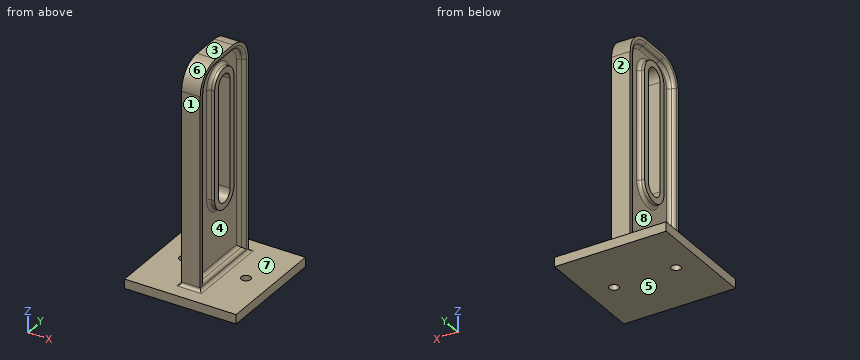
from build123d import *

# Parameters (mm, degrees)
SKETCH1_W           = 36
SKETCH1_H           = 36
BOSS_EXTRUDE1_DEPTH = 1.5
SKETCH2_R           = 1.5
CUT_EXTRUDE1_DEPTH  = 26.632011236
SKETCH3_W           = 6
SKETCH3_H           = 25
BOSS_EXTRUDE2_DEPTH = 70
CUT_EXTRUDE2_DEPTH  = 77.66322456
FILLET1_R           = 8
CUT_EXTRUDE3_DEPTH  = 2
FILLET4_R           = 1


with BuildPart() as part:
    # Sketch1 → Boss-Extrude1 (new, symmetric)
    with BuildSketch(Plane.XY):
        Rectangle(SKETCH1_W, SKETCH1_H)
    extrude(amount=BOSS_EXTRUDE1_DEPTH, both=True)

    # Sketch2 → Cut-Extrude1 (cut, through all)
    with BuildSketch(Plane.XY.offset(1.5)):
        with Locations((-10, 0)):
            Circle(SKETCH2_R)
        with Locations((10, 0)):
            Circle(SKETCH2_R)
    extrude(amount=-CUT_EXTRUDE1_DEPTH, mode=Mode.SUBTRACT)

    # Sketch3 → Boss-Extrude2 (add)
    with BuildSketch(Plane.XY.offset(1.5)):
        Rectangle(SKETCH3_W, SKETCH3_H)
    extrude(amount=BOSS_EXTRUDE2_DEPTH)

    # Sketch4 → Cut-Extrude2 (cut, through all)
    with BuildSketch(Plane(origin=(3, 0, 0), x_dir=(0, 0, -1), z_dir=(1, 0, 0))):
        with BuildLine():
            Line((-61.5, 3), (-26.5, 3))
            ThreePointArc((-26.5, 3), (-23.5, 0), (-26.5, -3))
            Line((-26.5, -3), (-61.5, -3))
            ThreePointArc((-61.5, -3), (-64.5, 0), (-61.5, 3))
        make_face()
    extrude(amount=-CUT_EXTRUDE2_DEPTH, mode=Mode.SUBTRACT)

    # Fillet1
    fillet1_edges = [part.edges().sort_by_distance(p)[0] for p in [
        (0, 12.5, 71.5),
        (0, -12.5, 71.5),
    ]]
    fillet(fillet1_edges, radius=FILLET1_R)

    # Sketch5 → Cut-Extrude3 (cut)
    with BuildSketch(Plane(origin=(3, 0, 0), x_dir=(0, 0, -1), z_dir=(1, 0, 0))):
        with BuildLine():
            Line((-3.5, -10.5), (-3.5, 10.5))
            Line((-3.5, 10.5), (-63.5, 10.5))
            ThreePointArc((-63.5, 10.5), (-67.742640687, 8.742640687), (-69.5, 4.5))
            Line((-69.5, 4.5), (-69.5, -4.5))
            ThreePointArc((-69.5, -4.5), (-67.742640687, -8.742640687), (-63.5, -10.5))
            Line((-63.5, -10.5), (-3.5, -10.5))
        make_face()
        with BuildLine():
            Line((-26.5, 5), (-61.5, 5))
            ThreePointArc((-61.5, 5), (-66.5, 0), (-61.5, -5))
            Line((-61.5, -5), (-26.5, -5))
            ThreePointArc((-26.5, -5), (-21.5, 0), (-26.5, 5))
        make_face(mode=Mode.SUBTRACT)
    cut_extrude3 = extrude(amount=-CUT_EXTRUDE3_DEPTH, mode=Mode.SUBTRACT)

    # Mirror1: Cut-Extrude3 across plane
    add(cut_extrude3.mirror(Plane(origin=(0, 0, 0), x_dir=(0, 0, 1), z_dir=(1, 0, 0))), mode=Mode.SUBTRACT)

    # Fillet4
    fillet4_edges = [part.edges().sort_by_distance(p)[0] for p in [
        (-3, -10.5, 33.5),
        (-3, -8.742640687, 67.742640687),
        (-3, 0, 69.5),
        (-3, 8.742640687, 67.742640687),
        (3, 10.5, 33.5),
        (3, 8.742640687, 67.742640687),
        (3, 0, 69.5),
        (3, -8.742640687, 67.742640687),
        (-1, 10.5, 33.5),
        (-1, 8.742640687, 67.742640687),
        (-1, 0, 69.5),
        (-1, -8.742640687, 67.742640687),
        (-1, -5, 44),
        (-1, 0, 66.5),
        (-1, 5, 44),
        (1, 10.5, 33.5),
        (1, 8.742640687, 67.742640687),
        (1, 0, 69.5),
        (1, -8.742640687, 67.742640687),
        (1, 0, 21.5),
        (1, -5, 44),
        (1, 0, 66.5),
        (0, 12.5, 1.5),
        (0, -12.5, 1.5),
        (-3, 0, 1.5),
        (3, 0, 1.5),
        (-3, 10.5, 33.5),
        (-3, 0, 3.5),
        (3, 0, 3.5),
        (3, -10.5, 33.5),
        (-1, 0, 3.5),
        (-1, -10.5, 33.5),
        (-1, 0, 21.5),
        (1, 0, 3.5),
        (1, -10.5, 33.5),
        (1, 5, 44),
    ]]
    fillet(fillet4_edges, radius=FILLET4_R - 0.0001)  # a hair under: the kernel refuses the full size


solid = part.part
Could you check a few things on this model? Use its own coordinates, in mm. Face numbers are marked on the shaded views. A direction names the side the tool comes from. Give positions to 0.01 mm unless a question says otherwise; leave off trailing zeros. Order: outer loops, then holes, each group sorted by start corner. A loop starts at its lowest first (then second) coordinate and runs counter-clockwise, first axis right, second up. Notation, with made-up numbers: (84.25, 7) - (105.25, 7) arc R23 cw to (105.25, 31) - close; hole circle Ø7 at (1, -30.5). An arc over 180 degrees is marked (long way). One line per item, written item: value. Start each with the question number.
1. Thinking about a two-plate mould opening in Y: for the marked faces 6, 7 and 8, which applies, +Y half, -Y half, draft (parallel to the pull), parting line (faces both ways), or undercut?
2. Imagine slicing it at A-A on x = 10. List the corners of the cut face in (y, z) for me.
3. For P1, Ø12, axis at x = -12, z = 64, coming from the -Y side; P2, Ø5, axis at x = -1, z = 47, coming from the -Y side; P3, Ø8, axis at y = -5, z = 39, coming from the +X side; P4, Ø12.5, axis at y = 0.5, z = 49.5, coming from the -X side, each with a flat end and sliding along its axis, tell me the tip position at first contact or that it passes through.
4. Imagine slicing it at D-D on y = 15.5. List the corners of the cut face in (x, z) for me, plus the area to 3 significant figures.
5. If I drill on probe 1 along Y at (x, z) = (10, 0.7); probe 2 along Y at (x, z) = (0.5, 35); probe 3 along Z at (x, y) = (-1.5, 16.5), over which ranges is the centre line in solid material (lowest first)?
6. For the marked faces 1, 2, 3, 4 and 5, which set-ups out of +Z, -Z, +X, -X, +Y, -Y let a thin tool reach every point of the face, with its end or its side?
7. Imagine slicing it at C-C on y = 0. Give the number of separate pieces and of enclosed holes in the cut face, plus the area to 3 significant figures.
Values:
1. face 6: -Y half
1. face 7: draft
1. face 8: undercut
2. outline: (-18, -1.5) - (-1.5, -1.5) - (-1.5, 1.5) - (-18, 1.5) - close; (1.5, -1.5) - (18, -1.5) - (18, 1.5) - (1.5, 1.5) - close
3. P1: through
3. P2: y = -12.5
3. P3: x = 3
3. P4: x = -3
4. outline: (-18, -1.5) - (18, -1.5) - (18, 1.5) - (-18, 1.5) - close
4. area: 108 mm²
5. probe 1: -18 to -1.5, 1.5 to 18
5. probe 2: -12.5 to -3, 3 to 12.5
5. probe 3: -1.5 to 1.5
6. face 1: +Z, +X, -X, -Y
6. face 2: +Z, +X, -X, +Y
6. face 3: +Z, +X, -X, +Y, -Y
6. face 4: +X
6. face 5: -Z, +X, -X, +Y, -Y
7. separate pieces: 4
7. enclosed holes: 0
7. area: 181 mm²
